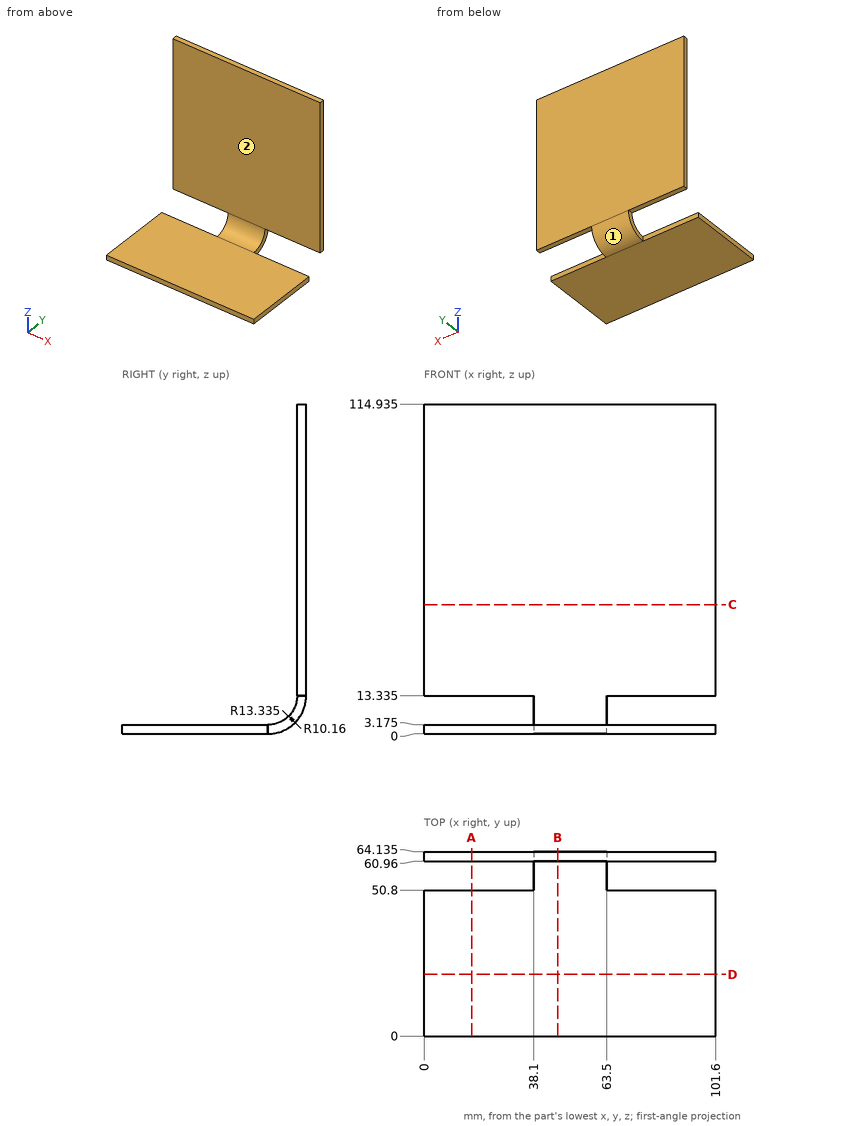
For this review, use the dimensioned drawing (mm, ordinates from the lowest corner) and the shaded views. A direction names the side the tool comes from. Coordinates: 2 decimals unless noted, no trailing zeros. Loops run counter-clockwise (first coordinate to the right, second up) from the corner with the lowest first, then second, coordinate; pieces in that order, holes last. Notation, with made-up numbers: (-25, 87) -> (3, 87) arc R9 cw to (3, 96) -> close; hole circle Ø2 at (5, -13). An arc over 180 degrees is marked (long way). Write each question's results on one line, items separated by ' | '.
Q1. Add section B-B, the plane x = 46.5. State the section outline as (y, z) points (3 decimals), then the cut area to 3 significant figures.
Taken from the geometry:
outline: (0, 0) -> (50.8, 0) arc R13.335 ccw to (64.135, 13.335) -> (64.135, 114.935) -> (60.96, 114.935) -> (60.96, 13.335) arc R10.16 cw to (50.8, 3.175) -> (0, 3.175) -> close | area: 542 mm²
Q2. Add section A-A, the plane x = 16.5. State the section outline as (y, z) points (3 decimals), then the cut area to 3 significant figures.
Taken from the geometry:
outline: (0, 0) -> (50.8, 0) -> (50.8, 3.175) -> (0, 3.175) -> close; (60.96, 13.335) -> (64.135, 13.335) -> (64.135, 114.935) -> (60.96, 114.935) -> close | area: 484 mm²
Q3. Add section C-C, the plane z = 45. State the section outline as (x, y) points (3 decimals).
Taken from the geometry:
outline: (0, 60.96) -> (101.6, 60.96) -> (101.6, 64.135) -> (0, 64.135) -> close
Q4. Add section D-D, the plane y = 21.5. State the section outline as (x, z) points (3 decimals).
Taken from the geometry:
outline: (0, 0) -> (101.6, 0) -> (101.6, 3.175) -> (0, 3.175) -> close
Q5. Machinability: for the marked faces 1 and 2, which of the approach directions +Z, -Z, +X, -X, +Y, -Y give a long, thin tool a straight path to every point of the face, cutting with its end or side? Answer none if there is none.
Taken from the geometry:
face 1: -Z, +X, -X, +Y | face 2: +Z, +X, -X, -Y
Q6. For pin 1 Ø4 at (y, z) = (58, 5.5) entering from -X; pin 2 Ø5 at (x, y) = (35, 30) entering from +Z (3 decimals); pin 3 Ø3.5 at (x, y) = (90.5, 62.5) entering from -Z (3 decimals), all flat-tipped, find the tip position at first contact; note any pin that passes through.
Taken from the geometry:
pin 1: x = 38.1 | pin 2: z = 3.175 | pin 3: z = 13.335
Q7. To check wall thickness, follow line 1 along Z through (x, y) = (77, 3.5) (3 decimals); line 2 along Y through (x, z) = (85.5, 15.5) (3 decimals); line 3 along Z through (x, y) = (49, 53). State the ranges of each line that lie inside material, in increasing order. Write a range as [from, to].
Taken from the geometry:
line 1: [0, 3.175] | line 2: [60.96, 64.135] | line 3: [0.18, 3.42]
